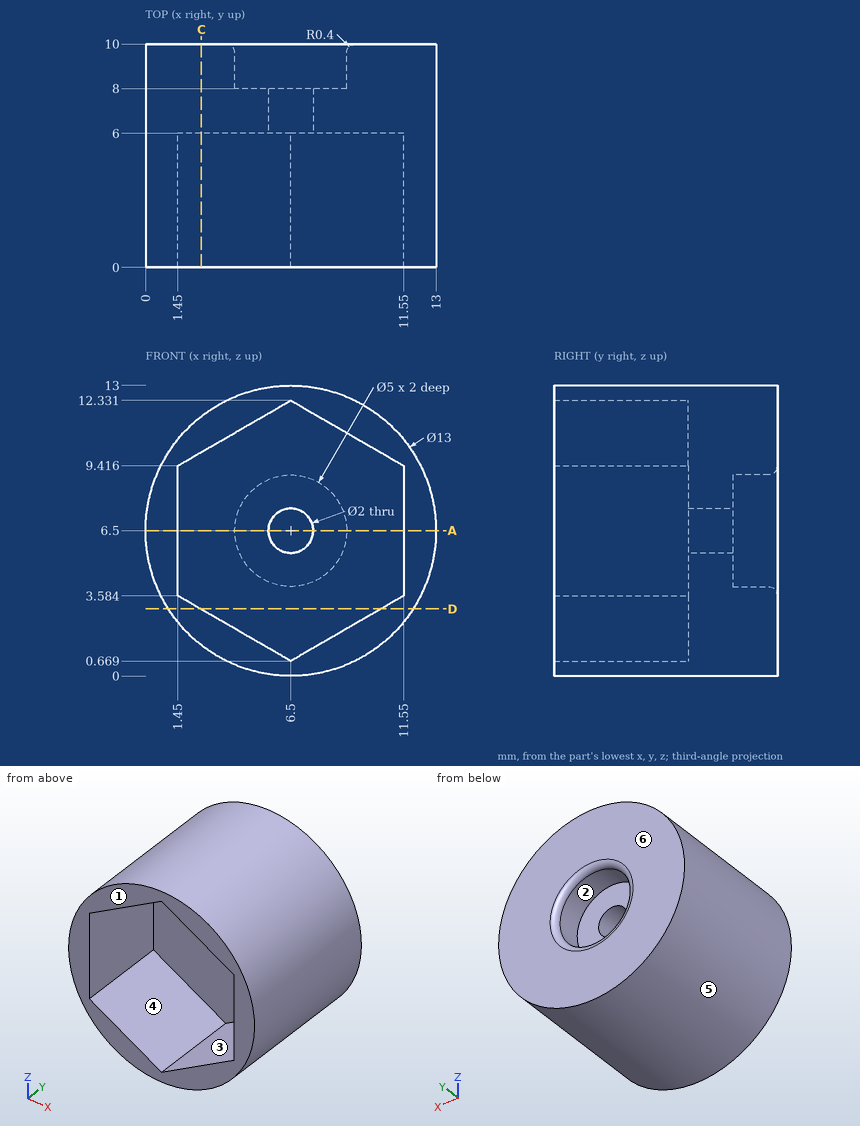
The drawing under review shows one solid part. Ordinate dimensions are in mm from its lowest x, y, z. A direction names the side the tool comes from. Round coordinates to 2 decimals unless told otherwise and drop trailing zeros. Loops run counter-clockwise (first coordinate to the right, second up) from the corner with the lowest first, then second, coordinate; pieces in that order, holes last. Notation, with made-up numbers: (-35, -28) -> (-21, -28) arc R32 ccw to (-21, 8) -> close; hole circle Ø1 at (-37, -14.5). An arc over 180 degrees is marked (long way). Answer in a Markdown table with one row per item.
1) Consider section A-A, the plane z = 6.5. Write out the cut boundary in (x, y).
Taken from the geometry:
| item | result |
|---|---|
| outline | (0, 0) -> (1.45, 0) -> (1.45, 6) -> (5.5, 6) -> (5.5, 8) -> (4, 8) -> (4, 9.6) arc R0.4 ccw to (3.6, 10) -> (0, 10) -> close; (7.5, 6) -> (11.55, 6) -> (11.55, 0) -> (13, 0) -> (13, 10) -> (9.4, 10) arc R0.4 ccw to (9, 9.6) -> (9, 8) -> (7.5, 8) -> close |
2) Consider section D-D, the plane z = 3. Write out the cut boundary in (x, y).
Taken from the geometry:
| item | result |
|---|---|
| outline | (1.02, 0) -> (2.46, 0) -> (2.46, 6) -> (10.54, 6) -> (10.54, 0) -> (11.98, 0) -> (11.98, 10) -> (1.02, 10) -> close |
3) Consider section C-C, the plane x = 2.5. Write out the cut boundary in (y, z).
Taken from the geometry:
| item | result |
|---|---|
| outline | (0, 1.38) -> (10, 1.38) -> (10, 11.62) -> (0, 11.62) -> (0, 10.02) -> (6, 10.02) -> (6, 2.98) -> (0, 2.98) -> close |
4) Draft analysis for pull direction X (two halves, no side actions). For the marked faces 4, 5 and 6, state which applies: pulls with the +X half, pulls with the -X half, needs draft (parallel to the pull), parting line crosses it, or undercut.
Taken from the geometry:
| item | result |
|---|---|
| face 4 | undercut |
| face 5 | parting line crosses it |
| face 6 | needs draft |
5) Wall thickness on line 1 along X through (y, z) = (6.75, 6.5); line 2 along X through (y, z) = (9.1, 6.5); line 3 along Y through (x, z) = (11.5, 4.75): over which ranges is each line inside the solid? List them lowest first.
Taken from the geometry:
| item | result |
|---|---|
| line 1 | x = 0 to 5.5, 7.5 to 13 |
| line 2 | x = 0 to 4, 9 to 13 |
| line 3 | y = 6 to 10 |
6) Tool access review of the marked faces 1, 2 and 3: name each direction out of +Z, -Z, +X, -X, +Y, -Y from which nothing blocks a thin tool from reaching the whole face with its end or side.
Taken from the geometry:
| item | result |
|---|---|
| face 1 | +Z, -Z, +X, -X, -Y |
| face 2 | +Y |
| face 3 | -Y |
7) For pin 1 Ø3 at (y, z) = (5.5, 1.5) entering from -X; pin 2 Ø1.6 at (x, z) = (6.5, 6.5) entering from -Y; pin 3 Ø1 at (y, z) = (5, 5.5) entering from +X; pin 4 Ø5 at (x, z) = (8.5, 7) entering from -Y, all flat-tipped, find the tip position at first contact; note any pin that passes through.
Taken from the geometry:
| item | result |
|---|---|
| pin 1 | stops at x = 1.02 |
| pin 2 | passes through |
| pin 3 | stops at x = 12.98 |
| pin 4 | stops at y = 6 |
